Verification items for this drawing (mm, ordinates from the low corner). Round coordinates to 2 decimals unless told otherwise and drop trailing zeros. Write each loop counter-clockwise with the first axis right and the second up, starting at its lowest first coordinate (ties: lowest second). Pieces come first, ordered by that corner, then holes.
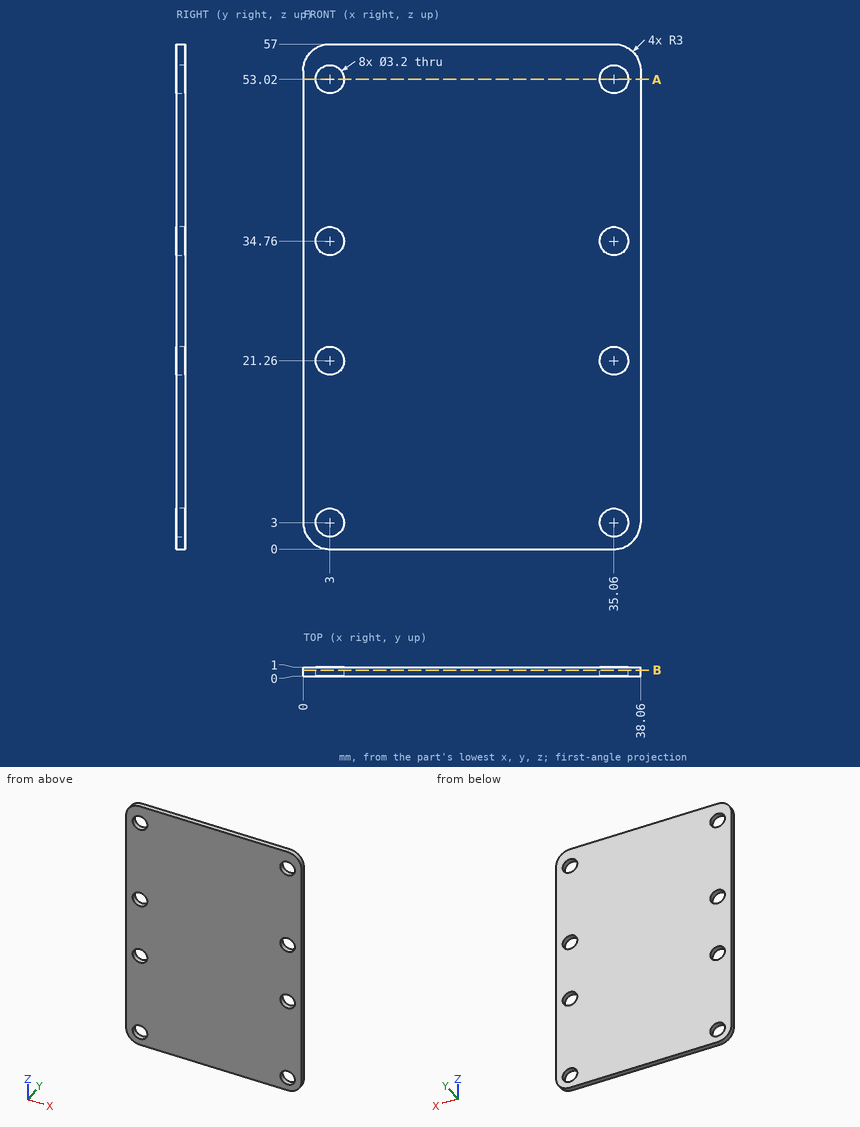
1. Scan line: line 1 along X through (y, z) = (0.8, 21.26). Record every from-to range of solid material in increasing order.
2. Depth check by flat-ended pin: pin 1 Ø3 at (x, z) = (35.06, 53.02) entering from -Y. Enter the tip coordinate at first touch or a pass-through.
3. Section check B-B (y = 0.65). State how many separate pieces and enclosed holes the cut face has, plus the area to 3 significant figures.
4. Section check A-A (z = 53.02). Record the cut outline in (x, y), plus the area to 3 significant figures.
Results below:
1. line 1: x = 0 to 1.4, 4.6 to 33.46, 36.66 to 38.06
2. pin 1: passes through
3. separate pieces: 1
3. enclosed holes: 8
3. area: 2,100 mm2
4. outline: (0, 0) - (1.4, 0) - (1.4, 1) - (0, 1) - close; (4.6, 0) - (33.46, 0) - (33.46, 1) - (4.6, 1) - close; (36.66, 0) - (38.06, 0) - (38.06, 1) - (36.66, 1) - close
4. area: 31.7 mm2
